Read the model definition and answer for the solid it produces. Units are mm, in the model's axes. A direction names the side the tool comes from. Give positions to 0.01 mm unless a question says otherwise; leave off trailing zeros. Order: outer loops, then holes, each group sorted by start corner. A loop starts at its lowest first (then second) coordinate and runs counter-clockwise, first axis right, second up. Notation, with made-up numbers: (18.25, -23) - (41.25, -23) arc R24 ccw to (41.25, -3) - close; hole circle Ø3 at (14.5, -29.5). An arc over 180 degrees is marked (long way). Write item = value, one per line.
```python
from build123d import *

# Parameters (mm, degrees)
F1_DEPTH = 3
F2_R     = 2
F3_DEPTH = 6
F4_R     = 2
F6_DEPTH = 12.5
F8_D     = 3
F9_R     = 0.99999


# Not quite as in the source:
# - a fillet or chamfer is up to 0.001 mm smaller than in the source, because OpenCascade refuses the exact size


with BuildPart() as f1:
    # F0 (on Front) → F1 (new body, symmetric)
    with BuildSketch(Plane.XZ):
        Polygon((0, 13), (0, 0), (7.5, 0), (7.5, 7), (14.5, 7), (14.5, 13), align=None)
    extrude(amount=F1_DEPTH, both=True)

    # F2 (on face) → F3 (join)
    with BuildSketch(Plane.XY.offset(13)):
        with Locations((11.5, 0)):
            Circle(F2_R)
    extrude(amount=F3_DEPTH)

    # F4
    f4_edges = [f1.edges().sort_by_distance(p)[0] for p in [
        (9.5, 0, 19),
    ]]
    fillet(f4_edges, radius=F4_R)

    # F5 (on Front) → F6 (cut, symmetric)
    with BuildSketch(Plane.XZ):
        with BuildLine():
            Line((10.7404427901, 17), (12.2404427901, 17))
            ThreePointArc((12.2404427901, 17), (11.4904427901, 17.75), (10.7404427901, 17))
        make_face()
        with BuildLine():
            ThreePointArc((10.7404427901, 17), (11.4904427901, 16.25), (12.2404427901, 17))
            Line((12.2404427901, 17), (10.7404427901, 17))
        make_face()
    extrude(amount=F6_DEPTH, both=True, mode=Mode.SUBTRACT)

    # F8 (through all)
    with Locations(Plane(origin=(0, 0, 0), x_dir=(1, 0, 0), z_dir=(0, 0, -1))):
        with Locations((3.3399870154, 0)):
            Hole(F8_D / 2)

    # F9 (radius 1 in the source; OpenCascade refuses exactly that, so slightly less here)
    f9_edges = [f1.edges().sort_by_distance(p)[0] for p in [
        (0, 3, 6.5),
        (7.25, 3, 13),
        (14.5, 3, 10),
        (11, 3, 7),
        (3.75, 3, 0),
        (7.5, 3, 3.5),
        (0, -3, 6.5),
        (7.5, -3, 3.5),
        (3.75, -3, 0),
        (7.25, -3, 13),
        (14.5, -3, 10),
        (0, 0, 13),
        (0, 0, 0),
        (7.5, 0, 0),
        (11, -3, 7),
        (14.5, 0, 13),
        (14.5, 0, 7),
    ]]
    fillet(f9_edges, radius=F9_R)


solid = f1.part
```
1. Section B-B (z = 5.75) is taken. Determine the outline of the cut face in (x, y).
Recorded:
outline = (0, -2) arc R1 ccw to (1, -3) - (6.5, -3) arc R1 ccw to (7.5, -2) - (7.5, 2) arc R1 ccw to (6.5, 3) - (1, 3) arc R1 ccw to (0, 2) - close; hole circle Ø3 at (3.34, 0)
2. Determine the mould class of faces 1 (the face through (10.049, -2.715, 7.301)), 2 (the face through (7.162, 2.699, 12.715)), 3 (the face through (14.215, -2.699, 10.028)), 4 (the face through (11.144, -0.028, 17.665)) for opening direction Z: +Z half, -Z half, draft (parallel to the pull), parting line (faces both ways), or undercut.
Recorded:
face_1 = -Z half
face_2 = +Z half
face_3 = draft
face_4 = undercut
3. Section D-D (x = 8.5) is taken. Determine the outline of the cut face in (y, z), and give its area (3 significant figures).
Recorded:
outline = (-3, 8) arc R1 ccw to (-2, 7) - (2, 7) arc R1 ccw to (3, 8) - (3, 12) arc R1 ccw to (2, 13) - (-2, 13) arc R1 ccw to (-3, 12) - close
area = 35.1 mm^2
4. Straight lines are drawn through the part: L1, parallel to X at y = 0, z = 17; L2, parallel to Z at x = 7.75, y = 2.1; L3, parallel to Z at x = 1.5, y = -0.9. For each, find the intervals that lie inside material, in ascending order. Write a range as [from, to].
Recorded:
L1 = [9.5, 10.74], [12.24, 13.5]
L2 = [7.01, 12.99]
L3 = [0, 13]
5. Section A-A (y = 0) is taken. Count the separate pieces of the cut face and the enclosed holes in it, and give its area (3 significant figures).
Recorded:
separate_pieces = 2
enclosed_holes = 1
area = 120 mm^2
6. Flat-ended cylindrical pins translate along their axes: pin 1 (1.2 mm diameter, centred on y = 0.5, z = 5.5, fed in from +X); pin 2 (3 mm diameter, centred on x = 4.5, y = -2, fed in from -Z); pin 3 (2 mm diameter, centred on x = 8.5, y = 0.5, fed in from +Z); pin 4 (1.2 mm diameter, centred on x = 10, y = 0, fed in from -Z). Find the tip coordinate at first contact, or state that the pin passes through.
Recorded:
pin_1 = 7.5
pin_2 = 0
pin_3 = 13
pin_4 = 7
7. For faces 5 (the face through (7.5, 0, 4)), 6 (the face through (12.423, -1.774, 14.972)), 7 (the face through (7.199, -2.715, 4.549)), 8 (the face through (7.199, 2.715, 4.549)), determine the directions among +Z, -Z, +X, -X, +Y, -Y from which every point of the face is accessible in a straight line to the end or side of a thin tool.
Recorded:
face_5 = -Z, +X, +Y, -Y
face_6 = +Z
face_7 = -Z, +X, -Y
face_8 = -Z, +X, +Y
